Here's the drawing with two shaded views (mm, measured from the low corner). I have some questions. Give positions to 0.01 mm unless a question says otherwise; leave off trailing zeros. Loops run counter-clockwise (first coordinate to the right, second up) from the corner with the lowest first, then second, coordinate; pieces in that order, holes last. Notation, with made-up numbers: (88, 74) - (109, 74) arc R27 cw to (109, 95) - close; hole circle Ø8 at (-16.75, -34.5). An arc over 180 degrees is marked (long way). Answer as a JSON object with one key per item and string values. Group by question number.
Item 1: Please list where these lines run through material, in increasing order: L1, parallel to X at y = 1.15, z = 23.5; L2, parallel to Z at x = 23, y = 1.65; L3, parallel to X at y = 0.85, z = 23.5.
Item 2: Suppose I cut it at A-A on x = 23.5. Write out the boundary of the cut face in (y, z).
Item 3: Suppose I cut it at C-C on z = 30.5. Write out the boundary of the cut face in (x, y), and give its area (3 significant figures).
Item 4: Suppose I cut it at B-B on z = 23.5. Write out the boundary of the cut face in (x, y), and give its area (3 significant figures).
Item 5: Will this pin go through, and if not, where does the flat tip stop? pin 1 (1 mm diameter, centred on y = 1, z = 24, fed in from -X).
Item 6: Suppose I cut it at D-D on y = 0.5. Write out the boundary of the cut face in (x, z).
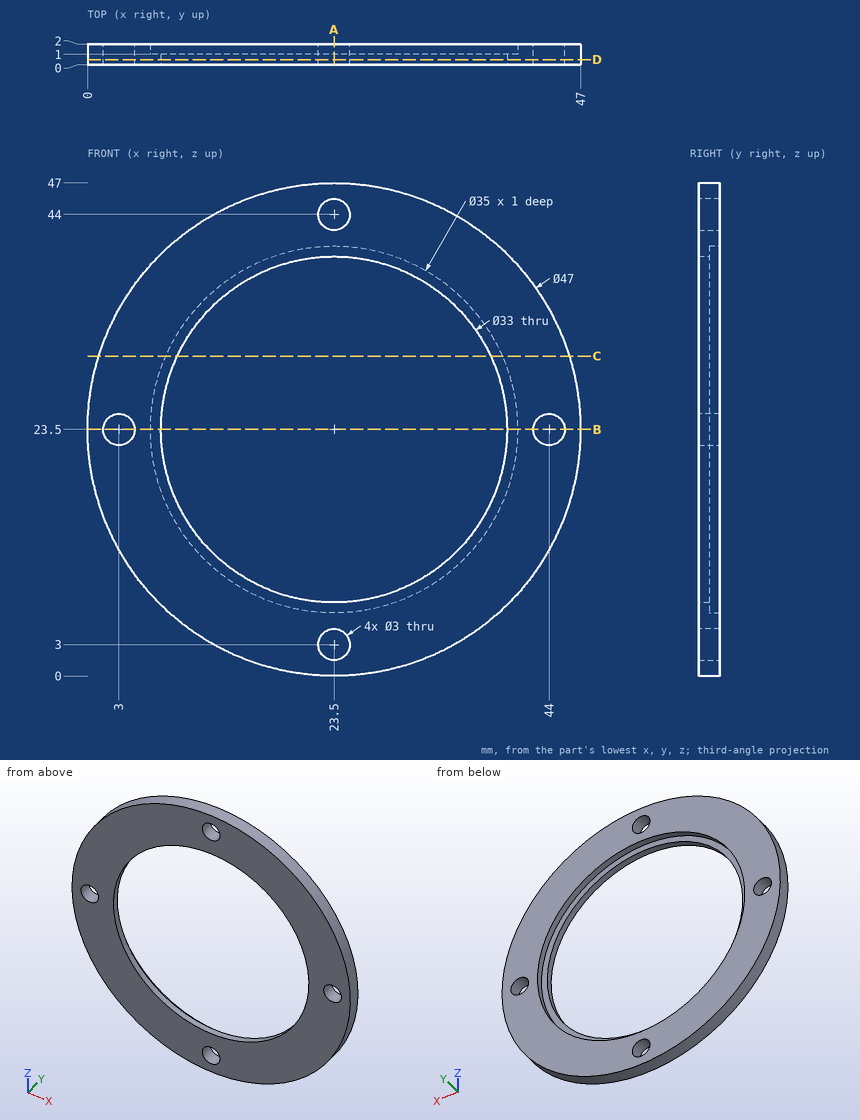
Worked out:
{
 "1": {"L1": "x = 0 to 1.5, 4.5 to 6, 41 to 42.5, 45.5 to 47", "L2": "z = 0.01 to 1.59, 4.41 to 6.01, 40.99 to 42.59, 45.41 to 46.99", "L3": "x = 0 to 1.5, 4.5 to 7, 40 to 42.5, 45.5 to 47"},
 "2": {"outline": "(0, 0) - (2, 0) - (2, 1.5) - (0, 1.5) - close; (0, 4.5) - (2, 4.5) - (2, 6) - (1, 6) - (1, 7) - (0, 7) - close; (0, 40) - (1, 40) - (1, 41) - (2, 41) - (2, 42.5) - (0, 42.5) - close; (0, 45.5) - (2, 45.5) - (2, 47) - (0, 47) - close"},
 "3": {"outline": "(1.07, 0) - (8.56, 0) - (8.56, 1) - (7.46, 1) - (7.46, 2) - (1.07, 2) - close; (38.44, 0) - (45.93, 0) - (45.93, 2) - (39.54, 2) - (39.54, 1) - (38.44, 1) - close", "area": "27.8 mm2"},
 "4": {"outline": "(0, 0) - (1.5, 0) - (1.5, 2) - (0, 2) - close; (4.5, 0) - (7, 0) - (7, 1) - (6, 1) - (6, 2) - (4.5, 2) - close; (40, 0) - (42.5, 0) - (42.5, 2) - (41, 2) - (41, 1) - (40, 1) - close; (45.5, 0) - (47, 0) - (47, 2) - (45.5, 2) - close", "area": "14.0 mm2"},
 "5": {"pin 1": "stops at x = 0"},
 "6": {"outline": "circle Ø47 at (23.5, 23.5); hole circle Ø3 at (3, 23.5); hole circle Ø33 at (23.5, 23.5); hole circle Ø3 at (23.5, 3); hole circle Ø3 at (23.5, 44); hole circle Ø3 at (44, 23.5)"}
}
